Here's how the part is built. I have some questions about the finished solid (model axes, mm). Face numbers are marked on the shaded views. A direction names the side the tool comes from. Round coordinates to 2 decimals unless told otherwise and drop trailing zeros. Loops run counter-clockwise (first coordinate to the right, second up) from the corner with the lowest first, then second, coordinate; pieces in that order, holes last. Notation, with made-up numbers: M -13,43 L 43,43 A32 ccw 43,76 Z; hole C 40,8.25 d6. An arc over 180 degrees is marked long. Answer as a JSON object with one key per item and string values.
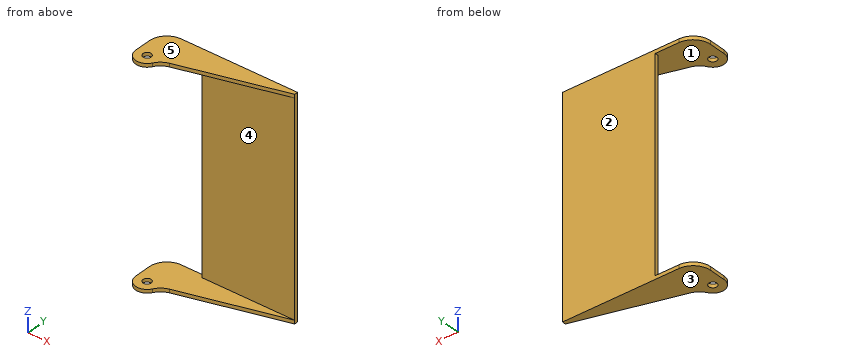
from build123d import *

# Parameters (mm, degrees)
SKETCH1_W               = 50
SKETCH1_H               = 123
BOSS_EXTRUDE1_DEPTH     = 2
BOSS_EXTRUDE2_DEPTH     = 123
CUT_EXTRUDE1_DEPTH      = 84.729178306
CUT_EXTRUDE1_DEPTH_BACK = 84.729178306
SKETCH3_W               = 119
SKETCH3_H               = 24.000498671
CUT_EXTRUDE2_DEPTH      = 85.324239069
CUT_EXTRUDE2_DEPTH_BACK = 85.324239069
SKETCH4_W               = 30.227049201
SKETCH4_H               = 119
CUT_EXTRUDE3_DEPTH      = 136.489207319
CUT_EXTRUDE3_DEPTH_BACK = 136.489207319
SKETCH5_R               = 2.3


with BuildPart() as part:
    # Sketch1 → Boss-Extrude1 (new body)
    with BuildSketch(Plane(origin=(0, 0, 0), x_dir=(1, 0, 0), z_dir=(0, 1, 0))):
        Rectangle(SKETCH1_W, SKETCH1_H)
    extrude(amount=BOSS_EXTRUDE1_DEPTH)

    # Sketch2 → Boss-Extrude2 (add)
    with BuildSketch(Plane.XY.offset(61.5)):
        with BuildLine():
            Line((-41.500498671, 2), (25, 2))
            Line((25, 2), (25, 0))
            Line((25, 0), (-33.350503344, -16.080973663))
            ThreePointArc((-33.350503344, -16.080973663), (-36.817369851, -17.815885758), (-39.363893872, -20.738949009))
            ThreePointArc((-39.363893872, -20.738949009), (-46.676153718, -23.780684014), (-51.500498671, -17.5))
            Line((-51.500498671, -17.5), (-51.500498671, -8))
            ThreePointArc((-51.500498671, -8), (-48.571566483, -0.928932188), (-41.500498671, 2))
        make_face()
    extrude(amount=-BOSS_EXTRUDE2_DEPTH)

    # Sketch3 → Cut-Extrude1 (cut, two sides: drawn at the far end of the back side and taken through both)
    with BuildSketch(Plane(origin=(0, 0, 0), x_dir=(0, 0, -1), z_dir=(1, 0, 0)).offset(-CUT_EXTRUDE1_DEPTH_BACK)):
        with Locations((0, -12.000249336)):
            Rectangle(SKETCH3_W, SKETCH3_H)
    extrude(amount=CUT_EXTRUDE1_DEPTH + CUT_EXTRUDE1_DEPTH_BACK, mode=Mode.SUBTRACT)

    # Sketch4 → Cut-Extrude2 (cut, two sides: drawn at the far end of the back side and taken through both)
    with BuildSketch(Plane(origin=(0, 2, 0), x_dir=(1, 0, 0), z_dir=(0, 1, 0)).offset(-CUT_EXTRUDE2_DEPTH_BACK)):
        with Locations((-43.1135246, 0)):
            Rectangle(SKETCH4_W, SKETCH4_H)
    extrude(amount=CUT_EXTRUDE2_DEPTH + CUT_EXTRUDE2_DEPTH_BACK, mode=Mode.SUBTRACT)

    # Sketch5 → Cut-Extrude3 (cut, two sides: drawn at the far end of the back side and taken through both)
    with BuildSketch(Plane.XY.offset(61.5).offset(-CUT_EXTRUDE3_DEPTH_BACK)):
        with Locations((-45, -17.5)):
            Circle(SKETCH5_R)
    extrude(amount=CUT_EXTRUDE3_DEPTH + CUT_EXTRUDE3_DEPTH_BACK, mode=Mode.SUBTRACT)


solid = part.part
Item 1: I'm going to push flat-ended pins straight in: pin 1 Ø1.6 at (y, z) = (1, 4.5) entering from -X; pin 2 Ø5.5 at (x, y) = (-45, -17.5) entering from +Z; pin 3 Ø12 at (x, z) = (-26, 36.5) entering from -Y. Where does each tip first touch, or does it pass through?
Resolved:
{"pin 1": "x = -28", "pin 2": "z = 61.5", "pin 3": "y = 0"}
Item 2: I want a section at B-B, the plane x = -45. Please give me the cut outline in (y, z).
Resolved:
{"outline": "M -24,-61.5 L -19.8,-61.5 L -19.8,-59.5 L -24,-59.5 Z; M -24,59.5 L -19.8,59.5 L -19.8,61.5 L -24,61.5 Z; M -15.2,-61.5 L 1.37,-61.5 L 1.37,-59.5 L -15.2,-59.5 Z; M -15.2,59.5 L 1.37,59.5 L 1.37,61.5 L -15.2,61.5 Z"}
Item 3: I want a section at A-A, the plane y = -11. Please give me the cut outline in (x, z), then the cut area to 3 significant figures.
Resolved:
{"outline": "M -51.5,-61.5 L -14.91,-61.5 L -14.91,-59.5 L -51.5,-59.5 Z; M -51.5,59.5 L -14.91,59.5 L -14.91,61.5 L -51.5,61.5 Z", "area": "146 mm²"}
Item 4: If we mould it in two halves opening along Z, with no side actions, what happens to the marked faces 1, 2 and 3? For each: pulls with the +Z half, pulls with the -Z half, needs draft (parallel to the pull), parting line crosses it, or undercut.
Resolved:
{"face 1": "undercut", "face 2": "needs draft", "face 3": "pulls with the -Z half"}
Item 5: Please list where these lines run through material, in increasing order: probe 1 along Z at (x, y) = (-37, -11); probe 2 along Y at (x, z) = (3, -1); probe 3 along X at (y, z) = (-17.5, 60.2). Write a range as from..to.
Resolved:
{"probe 1": "-61.5..-59.5, 59.5..61.5", "probe 2": "0..2", "probe 3": "-51.5..-47.3, -42.7..-36.39"}
Item 6: I want a section at D-D, the plane y = -2.5. Please give me the cut outline in (x, z), then the cut area to 3 significant figures.
Resolved:
{"outline": "M -49.85,-61.5 L 15.93,-61.5 L 15.93,-59.5 L -49.85,-59.5 Z; M -49.85,59.5 L 15.93,59.5 L 15.93,61.5 L -49.85,61.5 Z", "area": "263 mm²"}
Item 7: On a 3-axis mill with a long thin cutter (end or side, diameter ignored), from which of +Z, -Z, +X, -X, +Y, -Y can I reach the whole of each face in a straight line? I mean the marked faces 4 and 5. Say none if no direction works.
Resolved:
{"face 4": "+X, -X, -Y", "face 5": "+Z, +X, -X, +Y, -Y"}
Item 8: I want a section at C-C, the plane x = 19. Please give me the cut outline in (y, z).
Resolved:
{"outline": "M -1.65,-61.5 L 2,-61.5 L 2,61.5 L -1.65,61.5 L -1.65,59.5 L 0,59.5 L 0,-59.5 L -1.65,-59.5 Z"}
